Work out the finished part from the listing and answer in its coordinate system (mm). Coordinates: 2 decimals unless noted, no trailing zeros. Order: outer loops, then holes, each group sorted by start corner. A loop starts at its lowest first (then second) coordinate and runs counter-clockwise, first axis right, second up.
1. The part is cut by section A-A, the plane y = 0. Give the vertices of the cut face in (x, z) (3 decimals), then the cut area to 3 significant figures.
2. Flat-ended cylindrical pins translate along their axes: pin 1 Ø3 at (x, y) = (73.5, 0.5) entering from +Z; pin 2 Ø4.5 at (x, y) = (43.5, -0.5) entering from -Z; pin 3 Ø5.5 at (x, y) = (111.76, 0) entering from -Z; pin 4 Ø1.5 at (x, y) = (48.5, 2) entering from -Z. Find the tip coordinate at first contact, or state that the pin passes through.
3. The part is cut by section B-B, the plane z = 0. Give the vertices of the cut face in (x, y) (3 decimals), then the cut area to 3 significant figures.
4. Find the intervals of material crossed by probe 1 along Z at (x, y) = (86, 0) (3 decimals); probe 2 along Y at (x, z) = (152, 7), in increasing order.
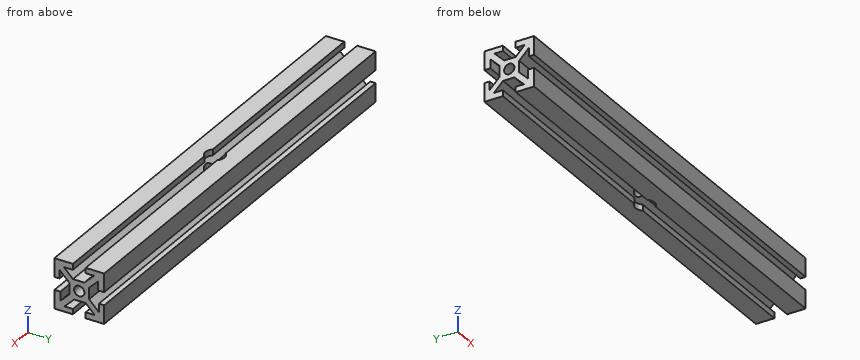
```python
from build123d import *

# Parameters (mm, degrees)
SKETCH1_W               = 10
SKETCH1_H               = 10
SKETCH1_R               = 2.605
BOSS_EXTRUDE1_DEPTH     = 223.52
CIRPATTERN1_COUNT       = 4
SKETCH2_R               = 4.765
CUT_EXTRUDE2_DEPTH      = 10
CUT_EXTRUDE2_DEPTH_BACK = 50


with BuildPart() as part:
    # Sketch1 → Boss-Extrude1 (new body)
    with BuildSketch(Plane(origin=(0, 0, 0), x_dir=(0, 0, -1), z_dir=(1, 0, 0))):
        Rectangle(SKETCH1_W, SKETCH1_H)
        Circle(SKETCH1_R, mode=Mode.SUBTRACT)
        Polygon((7.474873734, 9.921463197), (2.553410537, 5), (5, 5), (5, 3.203948776), (9.596194078, 7.800142853), align=None)
        Polygon((9.596194078, 3.24), (12.596194078, 3.24), (12.596194078, 12.596194078), (3.24, 12.596194078), (3.24, 9.921463197), (7.474873734, 9.921463197), (9.596194078, 7.800142853), align=None)
    boss_extrude1 = extrude(amount=BOSS_EXTRUDE1_DEPTH)

    # CirPattern1: Boss-Extrude1 ×4 about axis
    cirpattern1_axis = Axis((0, 0, 0), (1, 0, 0))
    for i in range(1, CIRPATTERN1_COUNT):
        add(boss_extrude1.rotate(cirpattern1_axis, i * 360 / CIRPATTERN1_COUNT))

    # Sketch2 → Cut-Extrude2 (cut, two sides)
    with BuildSketch(Plane.XY.offset(12.596194078)) as cut_extrude2_sk:
        with Locations((111.76, 0)):
            Circle(SKETCH2_R)
    extrude(amount=CUT_EXTRUDE2_DEPTH, mode=Mode.SUBTRACT)
    extrude(cut_extrude2_sk.sketch, amount=-CUT_EXTRUDE2_DEPTH_BACK, mode=Mode.SUBTRACT)


solid = part.part
```
Geometry says:
1. outline: (0, -5) - (106.995, -5) - (106.995, -2.605) - (0, -2.605) - close; (0, 2.605) - (106.995, 2.605) - (106.995, 5) - (0, 5) - close; (116.525, -5) - (223.52, -5) - (223.52, -2.605) - (116.525, -2.605) - close; (116.525, 2.605) - (223.52, 2.605) - (223.52, 5) - (116.525, 5) - close
1. area: 1,030 mm2
2. pin 1: stops at z = 5
2. pin 2: stops at z = -5.2
2. pin 3: passes through
2. pin 4: stops at z = -5
3. outline: (0, -5) - (223.52, -5) - (223.52, -2.605) - (115.75, -2.605) arc R4.765 cw to (107.77, -2.605) - (0, -2.605) - close; (0, 2.605) - (107.77, 2.605) arc R4.765 cw to (115.75, 2.605) - (223.52, 2.605) - (223.52, 5) - (0, 5) - close
3. area: 1,050 mm2
4. probe 1: z = -5 to -2.605, 2.605 to 5
4. probe 2: y = -12.6 to -9.92, -9.45 to -5.2, 4.55 to 8.8, 9.6 to 12.6
